Print and shaded views of the part. All mm, measured from the part's lowest x, y and z. A direction names the side the tool comes from. Give positions to 0.01 mm unless a question says otherwise; leave off trailing zeros. Order: outer loops, then holes, each group sorted by start corner. A loop starts at its lowest first (then second) coordinate and runs counter-clockwise, first axis right, second up. Notation, with made-up numbers: (78.5, -15) -> (86.5, -15) arc R6 cw to (86.5, -11) -> close; hole circle Ø6 at (25.5, 69). An arc over 180 degrees is marked (long way). One line per question, with ' | ' between items. Start each with the question number.
(1) Pin check, flat tips, straight feed: pin 1 Ø2 at (x, y) = (6, 5) entering from +Z; pin 2 Ø0.6 at (y, z) = (3, 3.5) entering from -X; pin 3 Ø3 at (x, y) = (1.5, 2) entering from -Z. Stop position of each tip, or through.
(2) Which spindle directions (+Z, -Z, +X, -X, +Y, -Y) get a long thin tool onto all of the face, cutting with end or side? Do the marked faces 4 and 5. Say none if no direction does.
(3) Pull direction Y, two halves, no side cores. Call the marked faces 1, 2 and 3: +Y half, -Y half, draft (parallel to the pull), parting line (faces both ways), or undercut.
(4) Cut at A-A (y = 3). Give the cut face in (x, z), then the cut area to 3 significant figures.
(5) Drill centre lines: L1, parallel to X at y = 2.75, z = 2.7; L2, parallel to X at y = 0.7, z = 1.8 (1 decimal); L3, parallel to Y at x = 0.75, z = 4.75 (1 decimal). Where is each one in solid material? Low to high. Write a range as from..to.
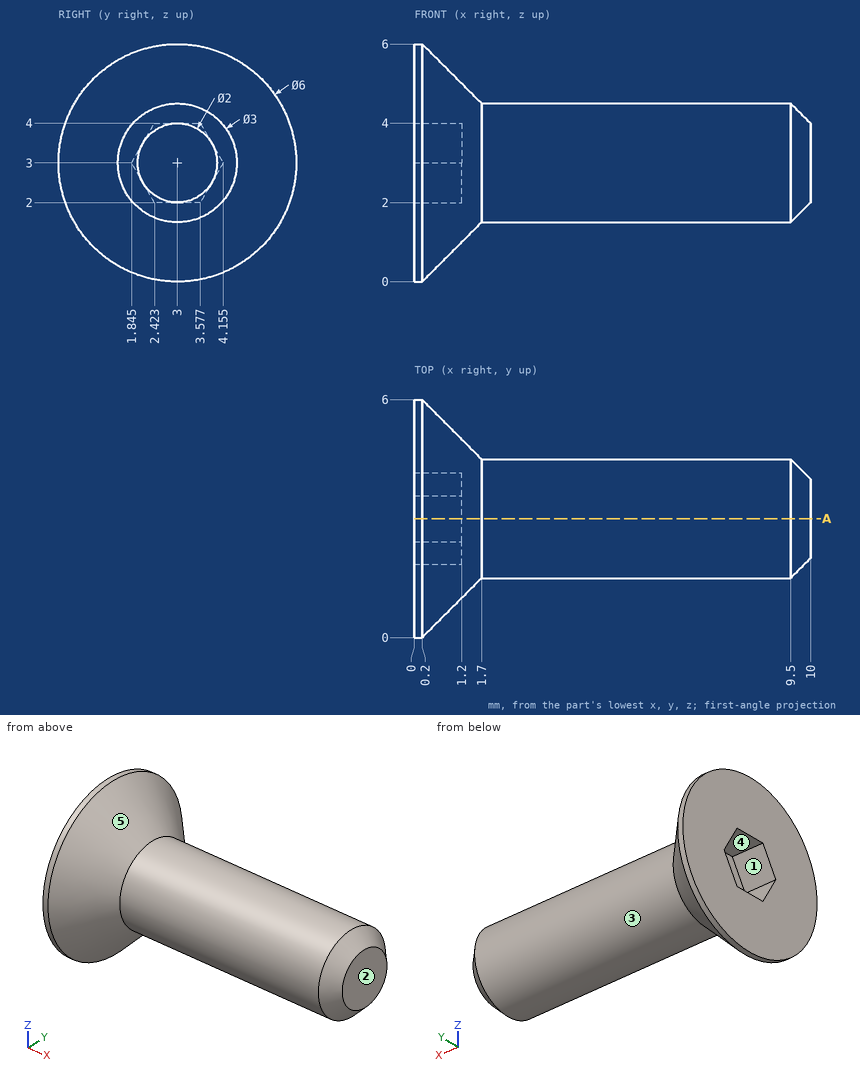
Result set:
1) pin 1: stops at z = 4.12 | pin 2: stops at x = 1.2 | pin 3: stops at z = 0.01
2) face 4: -X | face 5: +X
3) face 1: undercut | face 2: draft | face 3: parting line
4) outline: (0, 0) -> (0.2, 0) -> (1.7, 1.5) -> (9.5, 1.5) -> (10, 2) -> (10, 4) -> (9.5, 4.5) -> (1.7, 4.5) -> (0.2, 6) -> (0, 6) -> (0, 4) -> (1.2, 4) -> (1.2, 2) -> (0, 2) -> close | area: 30.2 mm2
5) L1: x = 1.2..10 | L2: x = 0..0.6 | L3: y = 1.3..4.7
